The model under review builds one solid part; all positions refer to its coordinate system, in mm. A direction names the side the tool comes from. Round coordinates to 2 decimals unless told otherwise and drop trailing zeros. Loops run counter-clockwise (first coordinate to the right, second up) from the corner with the lowest first, then second, coordinate; pieces in that order, holes last. Notation, with made-up numbers: (10.5, 75) - (39.5, 75) arc R5 cw to (39.5, 81) - close; hole circle Ø10 at (18, 45.5). An arc over 180 degrees is marked (long way). Answer as CSV lines item,"result".
from build123d import *

# Parameters (mm, degrees)
BOSS_EXTRUDE1_DEPTH = 6
SKETCH4_R           = 6
BOSS_EXTRUDE2_DEPTH = 6
SKETCH3_R           = 2
SKETCH3_R_2         = 6
CUT_EXTRUDE1_DEPTH  = 377.877964333


with BuildPart() as part:
    # Sketch2 → Boss-Extrude1 (new body)
    with BuildSketch(Plane(origin=(0, 0, 0), x_dir=(0, 0, -1), z_dir=(1, 0, 0))):
        Polygon((0, 376), (0, 0), (-25, 25), (-25, 351), align=None)
    extrude(amount=BOSS_EXTRUDE1_DEPTH)

    # Sketch4 → Boss-Extrude2 (add)
    with BuildSketch(Plane(origin=(6, 0, 0), x_dir=(0, 0, -1), z_dir=(1, 0, 0))):
        with Locations((-12, 364)):
            Circle(SKETCH4_R)
    extrude(amount=-BOSS_EXTRUDE2_DEPTH)

    # Sketch3 → Cut-Extrude1 (cut, through all)
    with BuildSketch(Plane(origin=(6, 0, 0), x_dir=(0, 0, -1), z_dir=(1, 0, 0))):
        with Locations((-12, 364)):
            Circle(SKETCH3_R)
        with Locations((-12, 12)):
            Circle(SKETCH3_R_2)
    extrude(amount=-CUT_EXTRUDE1_DEPTH, mode=Mode.SUBTRACT)


solid = part.part
1. Wall thickness on probe 1 along Y at (x, z) = (2.2, 12); probe 2 along Z at (x, y) = (4.45, 364); probe 3 along Y at (x, z) = (2.8, 7.5): over which ranges is each line inside the solid? List them lowest first.
Numbers:
probe 1,"y = 18 to 362, 366 to 370"
probe 2,"z = 0 to 10, 14 to 18"
probe 3,"y = 7.5 to 8.03, 15.97 to 368.5"
2. Take a section at B-B (y = 12). State the section outline as (x, z) points.
Numbers:
outline,"(0, 0) - (6, 0) - (6, 6) - (0, 6) - close"
3. Tool access review of faces 1 (the face through (3, 355, 21)), 2 (the face through (3, 191, 0)): name each direction out of +Z, -Z, +X, -X, +Y, -Y from which nothing blocks a thin tool from reaching the whole face with its end or side.
Numbers:
face 1,"+Z, +X, -X"
face 2,"-Z, +X, -X, +Y, -Y"
4. Draft analysis for pull direction Y (two halves, no side actions). For faces 3 (the face through (3.042, 368.335, 16.148)), 4 (the face through (3, 21, 21)), 5 (the face through (3, 372, 4)), 6 (the face through (0, 191, 12)), state which applies: +Y half, -Y half, draft (parallel to the pull), parting line (faces both ways), or undercut.
Numbers:
face 3,"undercut"
face 4,"-Y half"
face 5,"+Y half"
face 6,"draft"
5. Clearance check with a flat-ended pin moving along its axis: pin 1 (3 mm diameter, centred on x = 4.5, z = 12, fed in from +Y). State where the tip first meets the part, or that it passes through.
Numbers:
pin 1,"stops at y = 370"
6. Take a section at A-A (x = 2.5). State the section outline as (y, z) points, plus the area to 3 significant figures.
Numbers:
outline,"(0, 0) - (376, 0) - (368.24, 7.76) arc R6 ccw to (359.76, 16.24) - (351, 25) - (25, 25) - (16.24, 16.24) arc R6 cw to (7.76, 7.76) - close; hole circle Ø4 at (364, 12)"
area,"8,760 mm²"
